The model under review builds one solid part; all positions refer to its coordinate system, in mm. Face numbers are marked on the shaded views. A direction names the side the tool comes from. Coordinates: 2 decimals unless noted, no trailing zeros. Loops run counter-clockwise (first coordinate to the right, second up) from the corner with the lowest first, then second, coordinate; pieces in that order, holes last. Notation, with made-up numbers: M 62,84 L 81,84 A16 ccw 81,96 Z; hole C -22.5,-21.5 d2. An arc over 180 degrees is marked long. Use one line per item in the form item = value.
```python
from build123d import *

# Parameters (mm, degrees)
EXTRUDE_2_DEPTH     = 12
SKETCH_4_R          = 3
CUT_EXTRUDE_4_DEPTH = 29.861739379


with BuildPart() as part:
    # Эскиз2 → Вытянуть2 (new body)
    with BuildSketch(Plane.XY):
        Polygon((0.846446281, 0), (-29.153553719, 0), (-29.153553719, 4.760108812), (-19.153553719, 4.760108812), (-19.153553719, 17), (-9.153553719, 17), (-9.153553719, 4.760108812), (0.846446281, 4.760108812), align=None)
    extrude(amount=EXTRUDE_2_DEPTH)

    # Эскиз4 → Вытянуть4 (cut, through all)
    with BuildSketch(Plane.ZY.offset(19.153553719)):
        with Locations((6, 12.217021039)):
            Circle(SKETCH_4_R)
    extrude(amount=-CUT_EXTRUDE_4_DEPTH, mode=Mode.SUBTRACT)


solid = part.part
```
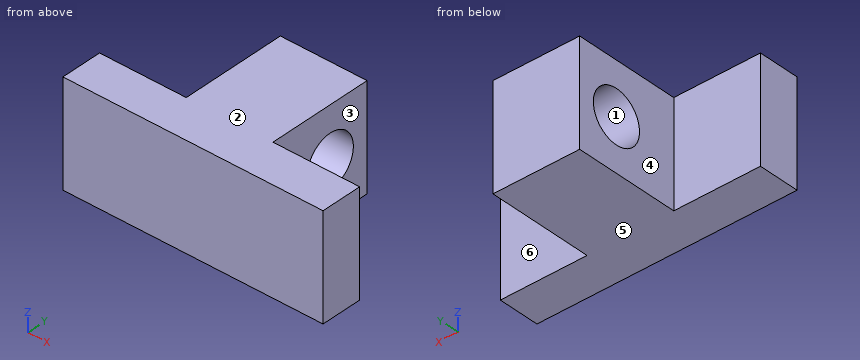
1. The part is to be moulded in two halves that separate along Z. For the marked faces 1, 2 and 3, say which applies: pulls with the +Z half, pulls with the -Z half, needs draft (parallel to the pull), parting line crosses it, or undercut.
Response values:
face_1 = undercut
face_2 = pulls with the +Z half
face_3 = needs draft
2. Add section A-A (z = 6). State the section outline as (x, y) points, then the cut area to 3 significant figures.
Response values:
outline = M -29.15,0 L 0.85,0 L 0.85,4.76 L -9.15,4.76 L -9.15,9.22 L -19.15,9.22 L -19.15,4.76 L -29.15,4.76 Z; M -19.15,15.22 L -9.15,15.22 L -9.15,17 L -19.15,17 Z
area = 205 mm^2
3. Add section C-C (z = 11). State the section outline as (x, y) points.
Response values:
outline = M -29.15,0 L 0.85,0 L 0.85,4.76 L -9.15,4.76 L -9.15,17 L -19.15,17 L -19.15,4.76 L -29.15,4.76 Z
4. Machinability: for the marked faces 4, 5 and 6, which of the approach directions +Z, -Z, +X, -X, +Y, -Y give a long, thin tool a straight path to every point of the face, cutting with its end or side? Answer none if there is none.
Response values:
face_4 = +Z, -Z, -X, +Y
face_5 = -Z, +X, -X, +Y, -Y
face_6 = +Z, -Z, +X, +Y
5. Wall thickness on line 1 along Y through (x, z) = (-15.25, 6); line 2 along Z through (x, y) = (-16, 10.5); line 3 along X through (y, z) = (9.25, 5): over which ranges is each line inside the solid? List them lowest first. Write a range as from..to.
Response values:
line_1 = 0..9.22, 15.22..17
line_2 = 0..3.54, 8.46..12
line_3 = -19.15..-9.15
6. Insertion check: P1, Ø5, axis at y = 12.22, z = 6, coming from the +X side. The pin has a flat end and moves straight along its axis. Give the tip position at first contact, or say it passes through.
Response values:
P1 = through
7. Add section D-D (x = -9.5). State the section outline as (y, z) points, then the cut area to 3 significant figures.
Response values:
outline = M 0,0 L 17,0 L 17,12 L 0,12 Z; hole C 12.22,6 d6
area = 176 mm^2
8. Add section B-B (y = 13.25). State the section outline as (x, z) points, then the cut area to 3 significant figures.
Response values:
outline = M -19.15,0 L -9.15,0 L -9.15,3.18 L -19.15,3.18 Z; M -19.15,8.82 L -9.15,8.82 L -9.15,12 L -19.15,12 Z
area = 63.7 mm^2
